Can you work these out from the model? Positions are in its coordinate system, mm. A direction names the side the tool comes from. Round coordinates to 2 decimals unless told otherwise and drop trailing zeros. Loops run counter-clockwise (first coordinate to the right, second up) from the corner with the lowest first, then second, coordinate; pieces in that order, holes last.
(1) I want a section at D-D on x = 2.5. Write out the boundary of the cut face in (y, z) (3 decimals), plus the area to 3 significant figures.
(2) I want a section at A-A on y = 0. Write out the boundary of the cut face in (x, z) (3 decimals).
(3) I want a section at C-C on x = 10. Write out the boundary of the cut face in (y, z) (1 decimal).
(4) I want a section at B-B on z = 2.65. Write out the boundary of the cut face in (x, y) (3 decimals).
(5) If I drill on line 1 along Y through (x, z) = (12.66, 1.5) (3 decimals); line 2 along X through (y, z) = (0.25, 5.3); line 3 along X through (y, z) = (1.5, 1.55), over which ranges is the centre line in solid material (lowest first)?
(6) Thinking about a two-plate mould opening in X: for faces 3 (the face through (5.66, -4, 3)), 4 (the face through (15.69, -0.95, 2.79)), 5 (the face through (9, -5.175, 3)), which applies, released by +X, released by -X, zero draft, split by the parting line, or undercut?
(7) Which directions (+Z, -Z, +X, -X, +Y, -Y) give clear straight access to the entire face, cutting with the end or side of a thin tool? Please do faces 1 (the face through (6, 5.175, 3)), 2 (the face through (3, -3.175, 3)).
(8) Will these pins go through, and if not, where does the flat tip stop? pin 1 Ø1.5 at (y, z) = (-2.5, 1.5) entering from +X; pin 2 Ø1.6 at (y, z) = (-4.5, 3.5) entering from -X; pin 3 Ø5 at (x, y) = (15.5, 0) entering from +Z.
Autodesk Inventor part; units mm, degrees
ref_plane "YZ Plane" through (0, 0, 0) normal (1, 0, 0) x (0, 1, 0)
ref_plane "XZ Plane" through (0, 0, 0) normal (0, 1, 0) x (-1, 0, 0)
ref_plane "XY Plane" through (0, 0, 0) normal (0, 0, 1) x (1, 0, 0)
sketch "Sketch1" plane through (0, 0, 0) normal (0, 0, 1) x (1, 0, 0)
  line L0 (0, 0) -> (0, -3.175)
  line L1 (0, -3.175) -> (5.16, -3.175)
  line L2 (0, 0) -> (0, 5.175)
  line L3 (0, 5.175) -> (12.66, 5.175)
  arc A0 (12.66, -5.175) -> (12.66, 5.175) centre (12.66, 0) ccw
  line L4 (12.66, -5.175) -> (5.66, -5.175)
  line L5 (5.66, -5.175) -> (5.66, -3.675)
  circle A1 centre (12.66, 0) radius 3.175
  arc A2 (5.66, -3.675) -> (5.16, -3.175) centre (5.66, -3.175) ccw
  dimension "d3" = 5.175
  dimension "d4" = 6.35
  dimension "d7" = 7
  dimension "d9" = 2
  dimension "d10" = 5.66
  dimension "d11" = 1
  dimension "d12" = 5.66
extrude "Extrusion1" add sketch "Sketch1" along normal blind 5.66
properties part number "Lower Arm Bracket"
Filled sheet:
1. outline: (-3.175, 0) - (5.175, 0) - (5.175, 5.66) - (-3.175, 5.66) - close
1. area: 47.3 mm2
2. outline: (0, 0) - (9.485, 0) - (9.485, 5.66) - (0, 5.66) - close; (15.835, 0) - (17.835, 0) - (17.835, 5.66) - (15.835, 5.66) - close
3. outline: (-5.2, 0) - (-1.7, 0) - (-1.7, 5.7) - (-5.2, 5.7) - close; (1.7, 0) - (5.2, 0) - (5.2, 5.7) - (1.7, 5.7) - close
4. outline: (0, -3.175) - (5.16, -3.175) arc R0.5 cw (long way) to (5.66, -3.675) - (5.66, -5.175) - (12.66, -5.175) arc R5.175 ccw to (12.66, 5.175) - (0, 5.175) - close; hole circle Ø6.35 at (12.66, 0)
5. line 1: y = -5.175 to -3.175, 3.175 to 5.175
5. line 2: x = 0 to 9.49, 15.83 to 17.83
5. line 3: x = 0 to 9.86, 15.46 to 17.61
6. face 3: released by -X
6. face 4: undercut
6. face 5: zero draft
7. face 1: +Z, -Z, +X, -X, +Y
7. face 2: +Z, -Z, -X, -Y
8. pin 1: stops at x = 17.53
8. pin 2: stops at x = 5.66
8. pin 3: stops at z = 5.66
